Print and shaded views of the part. All mm, measured from the part's lowest x, y and z. A direction names the side the tool comes from. Round coordinates to 2 decimals unless told otherwise and drop trailing zeros. Order: outer loops, then holes, each group sorted by start corner. A loop starts at its lowest first (then second) coordinate and runs counter-clockwise, first axis right, second up. Notation, with made-up numbers: (8.5, -7.5) -> (56.5, -7.5) arc R14 cw to (56.5, 12.5) -> close; hole circle Ø1 at (1, -19.5). An arc over 180 degrees is marked (long way). Answer as CSV lines item,"result".
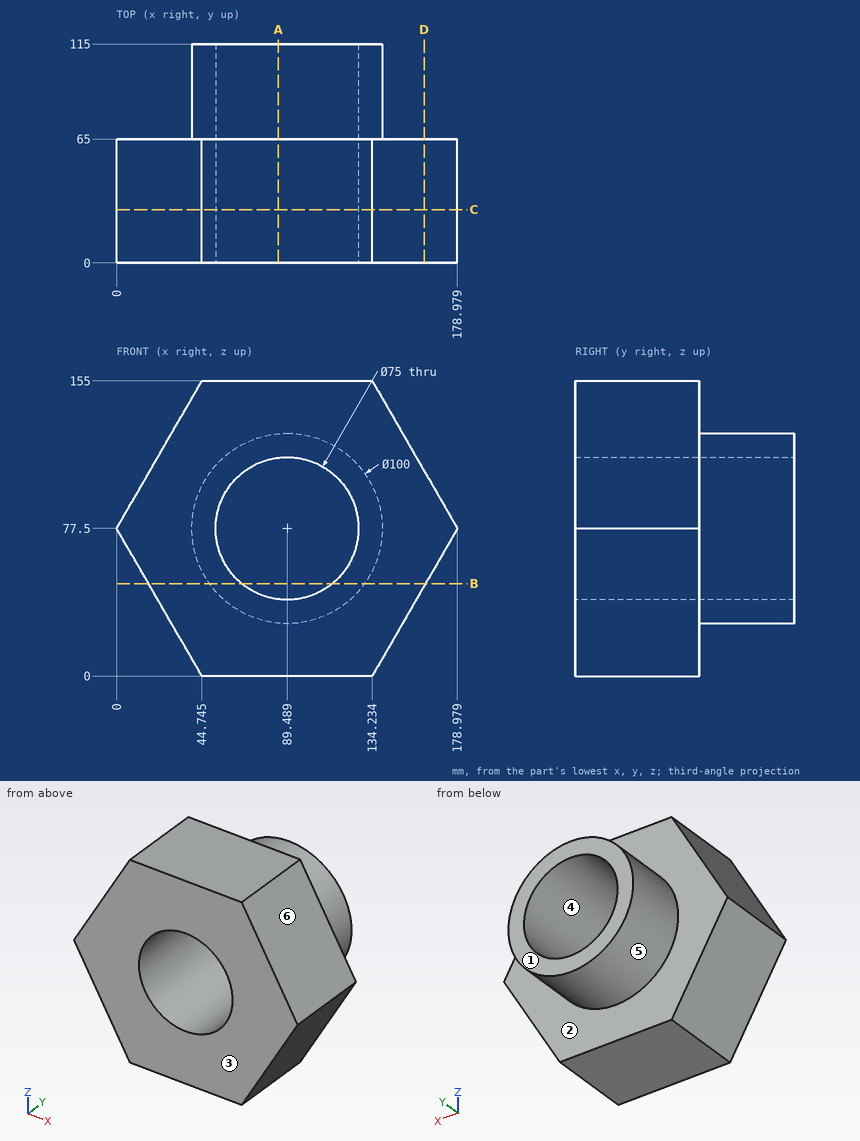
Q1. Saw through at B-B (z = 48.5). Write the cut outline in (x, y) (1 decimal), plus the area to 3 significant figures.
Checks:
outline,"(16.7, 0) -> (65.7, 0) -> (65.7, 115) -> (48.8, 115) -> (48.8, 65) -> (16.7, 65) -> close; (113.3, 0) -> (162.2, 0) -> (162.2, 65) -> (130.2, 65) -> (130.2, 115) -> (113.3, 115) -> close"
area,"8,060 mm²"
Q2. Saw through at C-C (y = 28). Write the cut outline in (x, z) (1 decimal), plus the area to 3 significant figures.
Checks:
outline,"(0, 77.5) -> (44.7, 0) -> (134.2, 0) -> (179, 77.5) -> (134.2, 155) -> (44.7, 155) -> close; hole circle Ø75 at (89.5, 77.5)"
area,"16,400 mm²"
Q3. Wall check: L1, parallel to X at y = 85, z = 77.5; L2, parallel to X at y = 52.5, z = 77.5; L3, parallel to Z at x = 63, y = 32 (1 decimal). Give the ranges that are in metal, low to high. Write a range as [from, to].
Checks:
L1,"[39.49, 51.99], [126.99, 139.49]"
L2,"[0, 51.99], [126.99, 178.98]"
L3,"[0, 51], [104, 155]"
Q4. Saw through at D-D (x = 161.5). Write the cut outline in (y, z), plus the area to 3 significant figures.
Checks:
outline,"(0, 47.23) -> (65, 47.23) -> (65, 107.77) -> (0, 107.77) -> close"
area,"3,940 mm²"
Q5. Mould opens along Z. For the marked faces 3, 4, 5 and 6 say: +Z half, -Z half, draft (parallel to the pull), parting line (faces both ways), or undercut.
Checks:
face 3,"draft"
face 4,"undercut"
face 5,"parting line"
face 6,"+Z half"
Q6. Tool access for the marked faces 1 and 2: list every direction of +Z, -Z, +X, -X, +Y, -Y with a clear straight run to the whole face (end or side of a thin tool).
Checks:
face 1,"+Z, -Z, +X, -X, +Y"
face 2,"+Y"
Q7. Flat gauge pins, fed straight in: pin 1 (1.5 mm diameter, centred on y = 24.5, z = 87, fed in from -X); pin 2 (10 mm diameter, centred on y = 48, z = 58.5, fed in from -X); pin 3 (8 mm diameter, centred on x = 77, y = 90.5, fed in from +Z). Where does each tip first touch, or does it go through?
Checks:
pin 1,"x = 5.05"
pin 2,"x = 8.08"
pin 3,"z = 126.77"
Q8. Saw through at A-A (x = 85). Write the cut outline in (y, z), plus the area to 3 significant figures.
Checks:
outline,"(0, 0) -> (65, 0) -> (65, 27.7) -> (115, 27.7) -> (115, 40.27) -> (0, 40.27) -> close; (0, 114.73) -> (115, 114.73) -> (115, 127.3) -> (65, 127.3) -> (65, 155) -> (0, 155) -> close"
area,"6,490 mm²"
